Autodesk Inventor part; units mm, degrees
ref_plane "YZ Plane" through (0, 0, 0) normal (1, 0, 0) x (0, 1, 0)
ref_plane "XZ Plane" through (0, 0, 0) normal (0, 1, 0) x (-1, 0, 0)
ref_plane "XY Plane" through (0, 0, 0) normal (0, 0, 1) x (1, 0, 0)
sketch "Esboço1" plane through (0, 0, 0) normal (0, 0, 1) x (1, 0, 0)
  circle A0 centre (0, 0) radius 0.8
  circle A1 centre (37.4, -29.1) radius 15.2
  line L0 (50.6, -101.1) -> (52.6, -101.1)
  line L1 (52.6, -101.1) -> (52.6, -45.7)
  line L2 (5.4, 7.4) -> (20.0215, 7.4)
  arc A2 (0, 7.4) -> (-7.2767, -1.3455) centre (0, 0) ccw
  line L3 (33.8, -29.1) -> (33.8, -2.8388)
  line L4 (31.3623, 1.4548) -> (22.5838, 6.6936)
  arc A3 (33.8, -37.1) -> (41, -37.1) centre (37.4, -37.1) ccw
  line L5 (33.8, -37.1) -> (33.8, -29.1)
  line L6 (37.4, -40.7) -> (47.6, -40.7)
  line L7 (0, 7.4) -> (7.6354, 7.4)
  line L8 (27.5941, -48.4938) -> (34.7764, -50.4183)
  line L9 (52.6, -101.1) -> (49.6, -101.1)
  line L10 (49.6, -101.1) -> (49.6, -69.7368)
  line L11 (52.6, -54.3903) -> (52.6, -101.1)
  arc A4 (49.6, -69.7368) -> (34.7764, -50.4183) centre (29.6, -69.7368) ccw
  arc A5 (52.6, -45.7) -> (47.6, -40.7) centre (47.6, -45.7) ccw
  arc A6 (22.5838, 6.6936) -> (20.0215, 7.4) centre (20.0215, 2.4) ccw
  arc A7 (33.8, -2.8388) -> (31.3623, 1.4548) centre (28.8, -2.8388) ccw
  line L12 (2, -101.1) -> (0, -101.1)
  line L13 (52.6, -51.1) -> (1.2194, -51.1) construction
  line L14 (25.0059, -48.4938) -> (17.8236, -50.4183)
  line L15 (0, -101.1) -> (3, -101.1)
  line L16 (3, -101.1) -> (3, -69.7368)
  arc A8 (17.8236, -50.4183) -> (3, -69.7368) centre (23, -69.7368) ccw
  circle A9 centre (0, 0) radius 7.4
  arc A10 (27.5941, -48.4938) -> (25.0059, -48.4938) centre (26.3, -53.3234) ccw
  line L17 (-7.4, 0) -> (-7.4, -101.1)
  line L18 (-7.4, -101.1) -> (0, -101.1)
  point P0 (21.4, 7.4)
  point P1 (49.6, -54.3903)
  point P2 (3, -54.3903)
  point P3 (49.5452, -41.9185)
  dimension "d7" = 20
  dimension "d9" = 5
  dimension "d11" = 5
extrude "Extrusão1" add sketch "Esboço1" against normal blind 3 contours L3 L5 A3 L6 A1 | A1 L6 A5 L1 L0 L9 L10 A4 L8 A10 L14 A8 L16 L15 L12 L18 L17 A2 A9 L7 L2 A6 L4 A7 L3 | A9 A2 picked at (30.2417, -33.5073)
properties part number "guarra"
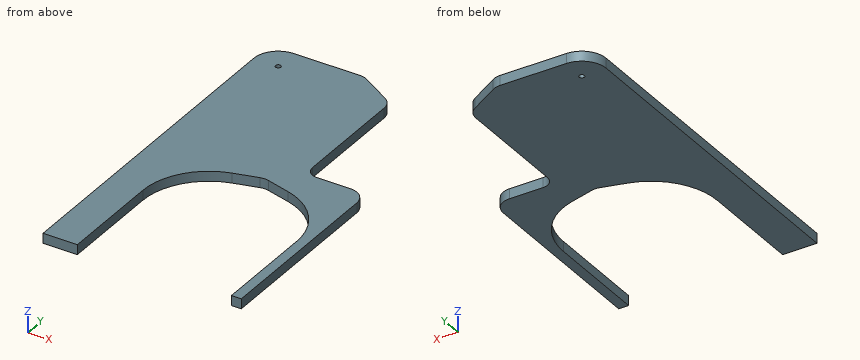
The listing builds one solid part. Answer for the finished solid, in the listing's coordinates (mm). Round coordinates to 2 decimals unless told otherwise and drop trailing zeros. Loops run counter-clockwise (first coordinate to the right, second up) from the corner with the lowest first, then second, coordinate; pieces in that order, holes last. Notation, with made-up numbers: (52, -14.5) -> (100, -14.5) arc R6 cw to (100, -6.5) -> close; hole circle Ø10 at (-14.5, 21). An arc over 180 degrees is marked (long way). Use one line per item in the form item = value.
1. A flat-ended cylindrical pin translates along its axis: pin 1 Ø1 at (y, z) = (-28.5, -2.5) entering from +X. Find the tip coordinate at first contact, or state that the pin passes through.
Answer key:
pin_1 = 33.8
2. Find the intervals of material crossed by probe 1 along X at (y, z) = (-76.5, -1.6); probe 2 along Y at (x, z) = (0, -1.15); probe 3 along X at (y, z) = (-58.5, -1.45), in increasing order. Write a range as [from, to].
Answer key:
probe_1 = [-7.4, 3], [49.6, 52.6]
probe_2 = [-101.1, -0.8], [0.8, 7.4]
probe_3 = [-7.4, 6.46], [46.14, 52.6]
3. The part is cut by section A-A on y = -78. Determine the outline of the cut face in (x, z).
Answer key:
outline = (-7.4, -3) -> (3, -3) -> (3, 0) -> (-7.4, 0) -> close; (49.6, -3) -> (52.6, -3) -> (52.6, 0) -> (49.6, 0) -> close
4. The part is cut by section C-C on x = 41. Determine the outline of the cut face in (y, z).
Answer key:
outline = (-53.3, -3) -> (-40.7, -3) -> (-40.7, 0) -> (-53.3, 0) -> close
5. The part is cut by section B-B on z = -1.75. Determine the outline of the cut face in (x, y), and give its area (3 significant figures).
Answer key:
outline = (-7.4, -101.1) -> (3, -101.1) -> (3, -69.74) arc R20 cw to (17.82, -50.42) -> (25.01, -48.49) arc R5 cw to (27.59, -48.49) -> (34.78, -50.42) arc R20 cw to (49.6, -69.74) -> (49.6, -101.1) -> (52.6, -101.1) -> (52.6, -45.7) arc R5 ccw to (47.6, -40.7) -> (37.4, -40.7) arc R3.6 cw to (33.8, -37.1) -> (33.8, -2.84) arc R5 ccw to (31.36, 1.45) -> (22.58, 6.69) arc R5 ccw to (20.02, 7.4) -> (0, 7.4) arc R7.4 ccw to (-7.4, 0) -> close; hole circle Ø1.6 at (0, 0)
area = 3,310 mm²
